Source: three-view drawing plus pictorial views. Frame: mm from the lowest corner of the part. Give positions to 0.01 mm unless a question says otherwise; leave off trailing zeros. Order: outer loops, then holes, each group sorted by start corner. A loop starts at its lowest first (then second) coordinate and runs counter-clockwise, first axis right, second up.
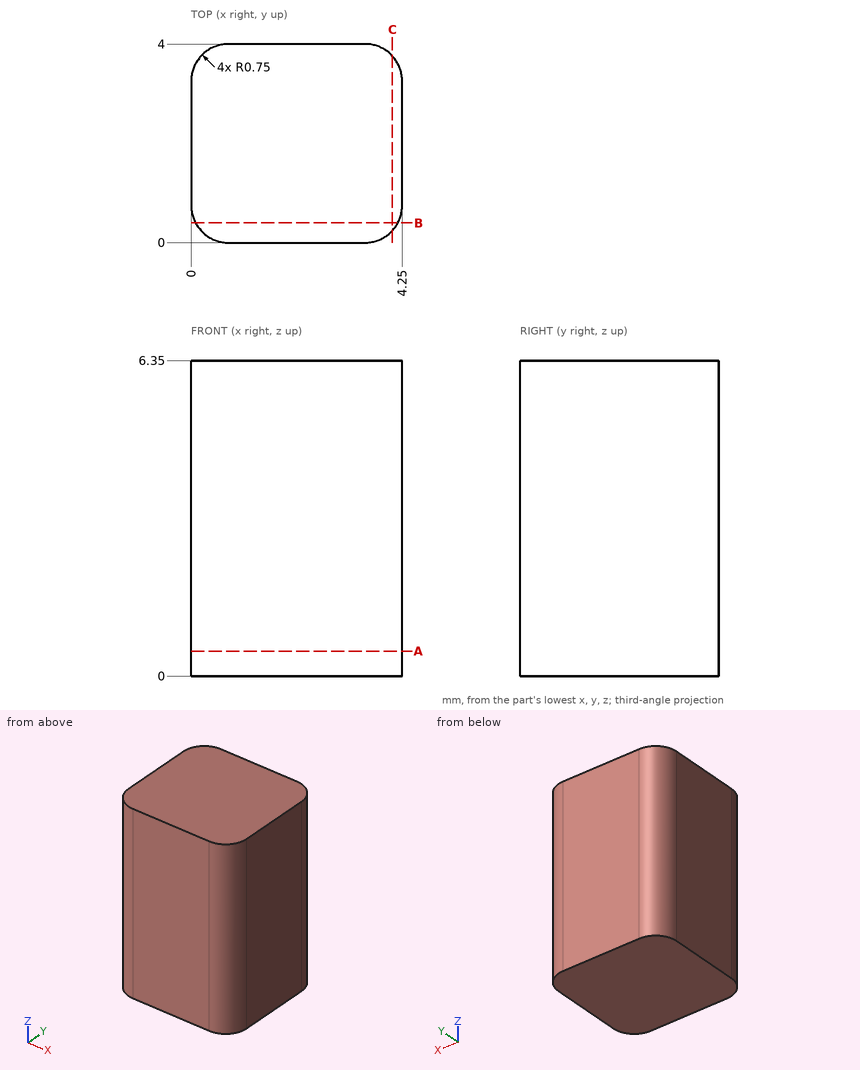
1) Section query C-C on x = 4.05. Output: boundary loops of the cut face in (y, z).
Checks:
outline: (0.24, 0) - (3.76, 0) - (3.76, 6.35) - (0.24, 6.35) - close
2) Ray query, L1, parallel to X at y = 0.7, z = 3; L2, parallel to Y at x = 3.8, z = 2.25; L3, parallel to Y at x = 0.2, z = 4.5. Return the intervals inside material, ascending.
Checks:
L1: x = 0 to 4.25
L2: y = 0.06 to 3.94
L3: y = 0.24 to 3.76
3) Section query A-A on z = 0.5. Output: boundary loops of the cut face in (x, y), and give its area (3 significant figures).
Checks:
outline: (0, 0.75) arc R0.75 ccw to (0.75, 0) - (3.5, 0) arc R0.75 ccw to (4.25, 0.75) - (4.25, 3.25) arc R0.75 ccw to (3.5, 4) - (0.75, 4) arc R0.75 ccw to (0, 3.25) - close
area: 16.5 mm2
4) Section query B-B on y = 0.4. Output: boundary loops of the cut face in (x, z), and give its area (3 significant figures).
Checks:
outline: (0.09, 0) - (4.16, 0) - (4.16, 6.35) - (0.09, 6.35) - close
area: 25.9 mm2
